Work out the finished part from the listing and answer in its coordinate system (mm). A direction names the side the tool comes from. Round coordinates to 2 decimals unless told otherwise and drop trailing zeros. Write each loop counter-clockwise with the first axis right and the second up, starting at its lowest first coordinate (ties: lowest second). Pieces come first, ordered by that corner, then holes. Notation, with made-up numbers: M 74,-29 L 127,-29 A27 cw 127,9 Z; hole C -10,78.25 d10. An arc over 180 degrees is marked long. Answer in a Markdown table with one row per item.
```python
from build123d import *

# Parameters (mm, degrees)
SKETCH1_W                = 190
SKETCH1_H                = 50
SKETCH1_W_2              = 140
SKETCH1_H_2              = 35
BOSS_EXTRUDE1_DEPTH      = 2
SKETCH3_W                = 190
SKETCH3_H                = 5
BOSS_EXTRUDE2_DEPTH      = 24
BOSS_EXTRUDE3_START      = -7.5
SKETCH6_W                = 5
SKETCH6_H                = 5.25
BOSS_EXTRUDE3_DEPTH      = 5.25
CUT_EXTRUDE1_DEPTH       = 108.905945309
SKETCH7_R                = 1.65
CUT_EXTRUDE2_DEPTH       = 5
FILLET1_R                = 2.75
FILLET1_OF_MIRROR3_R     = 2.75
CUT_EXTRUDE3_DEPTH       = 5
SKETCH10_W               = 6
SKETCH10_H               = 6
CUT_EXTRUDE4_DEPTH       = 1.6
CHAMFER1_SIZE            = 1
SKETCH12_W               = 6
SKETCH12_H               = 6
CUT_EXTRUDE5_DEPTH       = 1.6
CHAMFER1_OF_MIRROR5_SIZE = 1


with BuildPart() as part:
    # Sketch1 → Boss-Extrude1 (new body)
    with BuildSketch(Plane.XY):
        Rectangle(SKETCH1_W, SKETCH1_H)
        Rectangle(SKETCH1_W_2, SKETCH1_H_2, mode=Mode.SUBTRACT)
    extrude(amount=BOSS_EXTRUDE1_DEPTH)

    # Sketch3 → Boss-Extrude2 (add)
    with BuildSketch(Plane.XY.offset(2)):
        with Locations((0, 27.5)):
            Rectangle(SKETCH3_W, SKETCH3_H)
    extrude(amount=-BOSS_EXTRUDE2_DEPTH)

    # Sketch6 → Boss-Extrude3 (add)
    with BuildSketch(Plane.ZY.offset(95).offset(BOSS_EXTRUDE3_START)):
        with Locations((-17.5, 22.375)):
            Rectangle(SKETCH6_W, SKETCH6_H)
    boss_extrude3 = extrude(amount=-BOSS_EXTRUDE3_DEPTH)

    # Sketch5 → Cut-Extrude1 (cut, symmetric)
    with BuildSketch(Plane(origin=(0, 18.839521848, 4.396767931), x_dir=(1, 0, 0), z_dir=(0, 0.9738311486761368, 0.22727273014621918))):
        with BuildLine():
            Line((95, 28.242467175), (88.541117044, 28.242467175))
            ThreePointArc((88.541117044, 28.242467175), (91.551341518, 19.077417851), (95, 10.068181746))
            Line((95, 10.068181746), (95, 28.242467175))
        make_face()
    cut_extrude1 = extrude(amount=CUT_EXTRUDE1_DEPTH, both=True, mode=Mode.SUBTRACT)

    # Mirror1: Cut-Extrude1 across plane
    add(cut_extrude1.mirror(Plane(origin=(0, 0, 0), x_dir=(0, 0, 1), z_dir=(1, 0, 0))), mode=Mode.SUBTRACT)

    # Sketch7 → Cut-Extrude2 (cut)
    with BuildSketch(Plane(origin=(0, 0, -20), x_dir=(-1, 0, 0), z_dir=(0, 0, -1))):
        with Locations((84.875, 22.375)):
            Circle(SKETCH7_R)
    cut_extrude2 = extrude(amount=-CUT_EXTRUDE2_DEPTH, mode=Mode.SUBTRACT)

    # Fillet1
    # the kernel refuses this fillet: 2.75 mm, written as the material it takes off along each edge
    with BuildSketch(Plane(origin=(-87.5, 19.75, -8.125), x_dir=(0, 1, 0), z_dir=(0, 0, -1))) as fillet1_piece_1:
        with BuildLine():
            CenterArc((FILLET1_R, FILLET1_R), FILLET1_R, 180, 90)
            Line((0, FILLET1_R), (0, 0))
            Line((0, 0), (FILLET1_R, 0))
        make_face()
    extrude(amount=18.75, mode=Mode.SUBTRACT)
    with BuildSketch(Plane(origin=(-82.25, 19.75, -8.125), x_dir=(0, 1, 0), z_dir=(0, 0, -1))) as fillet1_piece_2:
        with BuildLine():
            CenterArc((FILLET1_R, -FILLET1_R), FILLET1_R, 90, 90)
            Line((0, -FILLET1_R), (0, 0))
            Line((0, 0), (FILLET1_R, 0))
        make_face()
    extrude(amount=18.75, mode=Mode.SUBTRACT)

    # Mirror3: Boss-Extrude3, Cut-Extrude2 across plane
    add(boss_extrude3.mirror(Plane(origin=(0, 0, 0), x_dir=(0, 0, 1), z_dir=(1, 0, 0))))
    add(cut_extrude2.mirror(Plane(origin=(0, 0, 0), x_dir=(0, 0, 1), z_dir=(1, 0, 0))), mode=Mode.SUBTRACT)

    # Fillet1 of Mirror3
    # the kernel refuses this fillet: 2.75 mm, written as the material it takes off along each edge
    with BuildSketch(Plane(origin=(87.5, 19.75, -8.125), x_dir=(0, 1, 0), z_dir=(0, 0, -1))) as fillet1_of_mirror3_piece_1:
        with BuildLine():
            CenterArc((FILLET1_OF_MIRROR3_R, -FILLET1_OF_MIRROR3_R), FILLET1_OF_MIRROR3_R, 90, 90)
            Line((0, -FILLET1_OF_MIRROR3_R), (0, 0))
            Line((0, 0), (FILLET1_OF_MIRROR3_R, 0))
        make_face()
    extrude(amount=18.75, mode=Mode.SUBTRACT)
    with BuildSketch(Plane(origin=(82.25, 19.75, -8.125), x_dir=(0, 1, 0), z_dir=(0, 0, -1))) as fillet1_of_mirror3_piece_2:
        with BuildLine():
            CenterArc((FILLET1_OF_MIRROR3_R, FILLET1_OF_MIRROR3_R), FILLET1_OF_MIRROR3_R, 180, 90)
            Line((0, FILLET1_OF_MIRROR3_R), (0, 0))
            Line((0, 0), (FILLET1_OF_MIRROR3_R, 0))
        make_face()
    extrude(amount=18.75, mode=Mode.SUBTRACT)

    # Sketch9 → Cut-Extrude3 (cut)
    with BuildSketch(Plane.XZ.offset(-25)):
        Polygon((-68.887905516, -22), (-71.387905516, -16), (-56.387905516, -16), (-58.887905516, -22), align=None)
    cut_extrude3 = extrude(amount=-CUT_EXTRUDE3_DEPTH, mode=Mode.SUBTRACT)

    # Mirror4: Cut-Extrude3 across plane
    add(cut_extrude3.mirror(Plane(origin=(0, 0, 0), x_dir=(0, 0, 1), z_dir=(1, 0, 0))), mode=Mode.SUBTRACT)

    # Sketch10 → Cut-Extrude4 (cut)
    with BuildSketch(Plane(origin=(0, 0, 0), x_dir=(-1, 0, 0), z_dir=(0, 0, -1))):
        with Locations((84.875, 22)):
            Rectangle(SKETCH10_W, SKETCH10_H)
    cut_extrude4 = extrude(amount=-CUT_EXTRUDE4_DEPTH, mode=Mode.SUBTRACT)

    # Chamfer1
    chamfer1_edges = [part.edges().sort_by_distance(p)[0] for p in [
        (-81.875, 22, 0),
        (-84.875, 19, 0),
        (-87.875, 22, 0),
    ]]
    chamfer(chamfer1_edges, length=CHAMFER1_SIZE)

    # Sketch12 → Cut-Extrude5 (cut)
    with BuildSketch(Plane(origin=(0, 0, 0), x_dir=(-1, 0, 0), z_dir=(0, 0, -1))):
        with Locations((-84.875, -22)):
            Rectangle(SKETCH12_W, SKETCH12_H)
    cut_extrude5 = extrude(amount=-CUT_EXTRUDE5_DEPTH, mode=Mode.SUBTRACT)

    # Mirror5: Cut-Extrude4, Cut-Extrude5 across plane
    add(cut_extrude4.mirror(Plane(origin=(0, 0, 0), x_dir=(0, 0, 1), z_dir=(1, 0, 0))), mode=Mode.SUBTRACT)
    add(cut_extrude5.mirror(Plane(origin=(0, 0, 0), x_dir=(0, 0, 1), z_dir=(1, 0, 0))), mode=Mode.SUBTRACT)

    # Chamfer1 of Mirror5
    chamfer1_of_mirror5_edges = [part.edges().sort_by_distance(p)[0] for p in [
        (81.875, 22, 0),
        (84.875, 19, 0),
        (87.875, 22, 0),
    ]]
    chamfer(chamfer1_of_mirror5_edges, length=CHAMFER1_OF_MIRROR5_SIZE)


solid = part.part
```
1. The part is cut by section B-B (y = -8.5). Determine the outline of the cut face in (x, z).
Calculated:
| item | result |
|---|---|
| outline | M -95,0 L -70,0 L -70,2 L -95,2 Z; M 70,0 L 95,0 L 95,2 L 70,2 Z |
2. A tool of negligible diameter and unlimited length cuts with its end or side. For faces 1 (the flat face through (86, 24, -15)), 2 (the cylindrical face through (83.66, 23.49, -17.54)), 3 (the flat face through (86, 24, -20)), 4 (the flat face through (-85, 22, 1.6)), 5 (the flat face through (64, 27, -16)), from which of +Z, -Z, +X, -X, +Y, -Y can it reach the whole face along a straight path? Write none if from no direction.
Calculated:
| item | result |
|---|---|
| face 1 | +X, -X, -Y |
| face 2 | -Z |
| face 3 | -Z, +X, -X, -Y |
| face 4 | none |
| face 5 | +Y, -Y |
3. Consider line 1 along X through (y, z) = (-21, 0.25) (3 decimals); line 2 along Y through (x, z) = (-39, -13.25); line 3 along Z through (x, y) = (-21.5, 23.5). Determine where each line is inside the solid, lowest interval first. Write a range as from..to.
Calculated:
| item | result |
|---|---|
| line 1 | x = -95..-87.875, -81.875..81.875, 87.875..95 |
| line 2 | y = 25..30 |
| line 3 | z = 0..2 |
4. The part is cut by section C-C (x = 64.5). Determine the outline of the cut face in (y, z), plus the area to 3 significant figures.
Calculated:
| item | result |
|---|---|
| outline | M -25,0 L -17.5,0 L -17.5,2 L -25,2 Z; M 17.5,0 L 25,0 L 25,-16 L 30,-16 L 30,2 L 17.5,2 Z |
| area | 120 mm² |
5. Given pin 1 (6 mm diameter, centred on x = 86, y = 21.5, fed in from -Z); pin 2 (0.8 mm diameter, centred on x = -86, z = 1, fed in from -Y); pin 3 (6.5 mm diameter, centred on x = 84.5, y = 23, fed in from -Z); pin 4 (8 mm diameter, centred on y = -1.5, z = -6.5, fed in from +X), each flat-ended and moving along its own axis, determine where each tip first touches the part or whether it passes through.
Calculated:
| item | result |
|---|---|
| pin 1 | stops at z = -20 |
| pin 2 | stops at y = -19 |
| pin 3 | stops at z = -22 |
| pin 4 | passes through |
6. The part is cut by section A-A (x = 10.5). Determine the outline of the cut face in (y, z), plus the area to 3 significant figures.
Calculated:
| item | result |
|---|---|
| outline | M -25,0 L -17.5,0 L -17.5,2 L -25,2 Z; M 17.5,0 L 25,0 L 25,-22 L 30,-22 L 30,2 L 17.5,2 Z |
| area | 150 mm² |
7. Determine the mould class of faces 6 (the flat face through (-95, 8.2, 0.2)), 7 (the cylindrical face through (-83.66, 23.49, -17.54)), 8 (the flat face through (-1, 28, -22)) for opening direction X: released by +X, released by -X, zero draft, split by the parting line, or undercut.
Calculated:
| item | result |
|---|---|
| face 6 | released by -X |
| face 7 | undercut |
| face 8 | zero draft |
